The listing builds one solid part. Answer for the finished solid, in the listing's coordinates (mm). A direction names the side the tool comes from. Coordinates: 2 decimals unless noted, no trailing zeros. Order: outer loops, then holes, each group sorted by start corner. A loop starts at its lowest first (then second) coordinate and runs counter-clockwise, first axis right, second up. Notation, with made-up numbers: (61.5, -17) -> (76.5, -17) arc R20 ccw to (76.5, 14) -> close; hole circle Ø3 at (-33, 38.5). An arc over 180 degrees is marked (long way). Return JSON: item names as keys, results as strings.
from build123d import *

# Parameters (mm, degrees)
SKETCH_R        = 20
PAD_DEPTH       = 3
POCKET_DEPTH    = 2.25
SKETCH002_R     = 3.907938
POCKET001_DEPTH = 2
SKETCH004_R     = 1
POCKET004_DEPTH = 5


with BuildPart() as part:
    # Sketch → Pad (new body)
    with BuildSketch(Plane.XY):
        Circle(SKETCH_R)
    extrude(amount=PAD_DEPTH)

    # Sketch001 (on Face3 of Pad) → Pocket (cut)
    with BuildSketch(Plane.XY.offset(3)):
        with BuildLine():
            ThreePointArc((1.890302, 3.525161), (0, 4.000122), (-1.890302, 3.525161))
            Line((-16.713594, 1.572988), (-1.890302, 3.525161))
            ThreePointArc((-16.713594, 1.572988), (-18.55, -0.42031), (-16.713594, -2.413609))
            Line((-16.713594, -2.413609), (-1.890302, -3.525161))
            ThreePointArc((-1.890302, -3.525161), (0, -3.996936), (1.890302, -3.525161))
            Line((1.890302, -3.525161), (16.713789, -2.411491))
            ThreePointArc((16.713789, -2.411491), (18.55, -0.418209), (16.713789, 1.575073))
            Line((1.890302, 3.525161), (16.713789, 1.575073))
        make_face()
    extrude(amount=-POCKET_DEPTH, mode=Mode.SUBTRACT)

    # Sketch002 (on Face12 of Pocket) → Pocket001 (cut)
    with BuildSketch(Plane.XY.offset(0.75)):
        Circle(SKETCH002_R)
    extrude(amount=-POCKET001_DEPTH, mode=Mode.SUBTRACT)

    # Sketch004 (on Face3 of Pocket001) → Pocket004 (cut)
    with BuildSketch(Plane.XY.offset(3)):
        with Locations((-10, 10)):
            Circle(SKETCH004_R)
        with Locations((10, 10)):
            Circle(SKETCH004_R)
        with Locations((10, -10)):
            Circle(SKETCH004_R)
        with Locations((-10, -10)):
            Circle(SKETCH004_R)
    extrude(amount=-POCKET004_DEPTH, mode=Mode.SUBTRACT)


solid = part.part
1. The part is cut by section A-A on y = 0. Give the vertices of the cut face in (x, z), and give its area (3 significant figures).
Answer block:
{"outline": "(-20, 0) -> (-3.91, 0) -> (-3.91, 0.75) -> (-18.51, 0.75) -> (-18.51, 3) -> (-20, 3) -> close; (3.91, 0) -> (20, 0) -> (20, 3) -> (18.51, 3) -> (18.51, 0.75) -> (3.91, 0.75) -> close", "area": "30.9 mm2"}
2. Determine the mould class of faces 3 (the face through (10, 11, 2)), 4 (the face through (4.2, 0.3, 0)), 5 (the face through (-10, 11, 2)), 6 (the face through (-4.336, -19.524, 1.479)) for opening direction X: pulls with the +X half, pulls with the -X half, needs draft (parallel to the pull), parting line crosses it, or undercut.
Answer block:
{"face 3": "undercut", "face 4": "needs draft", "face 5": "undercut", "face 6": "parting line crosses it"}
3. The part is cut by section D-D on x = -3. Give the vertices of the cut face in (y, z).
Answer block:
{"outline": "(-19.77, 0) -> (-2.5, 0) -> (-2.5, 0.75) -> (-3.44, 0.75) -> (-3.44, 3) -> (-19.77, 3) -> close; (2.5, 0) -> (19.77, 0) -> (19.77, 3) -> (3.38, 3) -> (3.38, 0.75) -> (2.5, 0.75) -> close"}
4. The part is cut by section B-B on z = 2. Give the vertices of the cut face in (x, y).
Answer block:
{"outline": "circle Ø40 at (0, 0); hole (-16.71, -2.41) -> (-1.89, -3.53) arc R4.02 ccw to (1.89, -3.53) -> (16.71, -2.41) arc R2 ccw to (16.71, 1.58) -> (1.89, 3.53) arc R4 ccw to (-1.89, 3.53) -> (-16.71, 1.57) arc R2 ccw to start; hole circle Ø2 at (-10, -10); hole circle Ø2 at (-10, 10); hole circle Ø2 at (10, -10); hole circle Ø2 at (10, 10)"}
5. The part is cut by section C-C on x = -10. Give the vertices of the cut face in (y, z).
Answer block:
{"outline": "(-17.32, 0) -> (-11, 0) -> (-11, 3) -> (-17.32, 3) -> close; (-9, 0) -> (9, 0) -> (9, 3) -> (2.46, 3) -> (2.46, 0.75) -> (-2.92, 0.75) -> (-2.92, 3) -> (-9, 3) -> close; (11, 0) -> (17.32, 0) -> (17.32, 3) -> (11, 3) -> close"}
6. This flat-tipped pin is pushed along its axis until it touches: pin 1 Ø2.5 at (x, y) = (-10, 10) entering from -Z. Where does it stop, or does it pass through?
Answer block:
{"pin 1": "stops at z = 0"}
7. For faces 1 (the face through (-10, -9, 2)), 2 (the face through (0, 4, 2)), determine the directions among +Z, -Z, +X, -X, +Y, -Y from which every point of the face is accessible in a straight line to the end or side of a thin tool.
Answer block:
{"face 1": "+Z, -Z", "face 2": "+Z"}
8. Consider line 1 (Y direction, x = 0, z = 0.65); line 2 (Y direction, x = 4, z = 1.95); line 3 (Z direction, x = 16, y = -0.5). Determine where each line is inside the solid, lowest interval first. Write a range as from..to.
Answer block:
{"line 1": "y = -20..-3.91, 3.91..20", "line 2": "y = -19.6..-3.37, 3.25..19.6", "line 3": "z = 0..0.75"}
